Verification items for the finished model (mm, model axes). Round coordinates to 2 decimals unless told otherwise and drop trailing zeros. Write each loop counter-clockwise with the first axis right and the second up, starting at its lowest first coordinate (ties: lowest second). Pieces come first, ordered by that corner, then holes. Notation, with made-up numbers: (12.5, -36.75) -> (42.5, -36.75) arc R14 cw to (42.5, -14.75) -> close; hole circle Ø11 at (-14.5, -2). An arc over 180 degrees is marked (long way). Use CSV: the item, a comma, the result in double quotes.
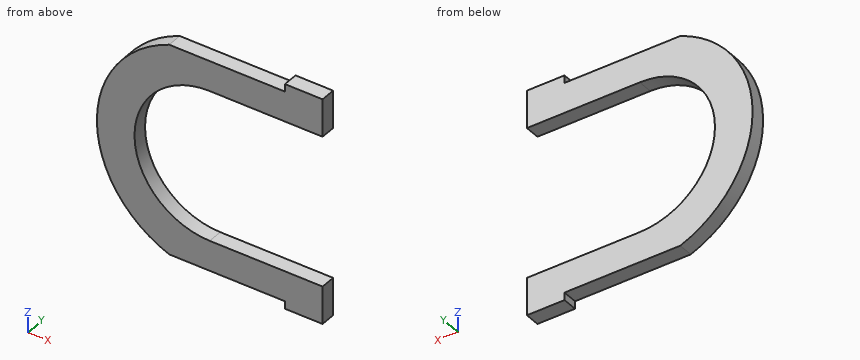
```python
from build123d import *

# Parameters (mm, degrees)
F1_DEPTH = 25.4


with BuildPart() as f1:
    # F0 (on Front) → F1 (new body)
    with BuildSketch(Plane.XZ):
        with BuildLine():
            Line((-68.391593, -177.8), (127, -177.8))
            Line((127, -177.8), (127, -190.5))
            Line((127, -190.5), (190.5, -190.5))
            Line((190.5, -190.5), (190.5, -177.8))
            Line((190.5, -177.8), (190.5, -127))
            Line((190.5, -127), (127, -127))
            Line((127, -127), (0, -127))
            ThreePointArc((0, -127), (-127, 0), (0, 127))
            Line((0, 127), (127, 127))
            Line((127, 127), (190.5, 127))
            Line((190.5, 127), (190.5, 177.8))
            Line((190.5, 177.8), (190.5, 190.5))
            Line((190.5, 190.5), (127, 190.5))
            Line((127, 190.5), (127, 177.8))
            Line((127, 177.8), (-68.391593, 177.8))
            ThreePointArc((-68.391593, 177.8), (-190.5, 0), (-68.391593, -177.8))
        make_face()
    extrude(amount=F1_DEPTH)


solid = f1.part
```
Q1. Section check C-C (z = 0). Record the cut outline in (x, y).
Filled in:
outline,"(-190.5, -25.4) -> (-127, -25.4) -> (-127, 0) -> (-190.5, 0) -> close"
Q2. Section check A-A (x = 122). Record the cut outline in (y, z), plus the area to 3 significant figures.
Filled in:
outline,"(-25.4, -177.8) -> (0, -177.8) -> (0, -127) -> (-25.4, -127) -> close; (-25.4, 127) -> (0, 127) -> (0, 177.8) -> (-25.4, 177.8) -> close"
area,"2,580 mm²"
Q3. Section check D-D (x = -17.5). Record the cut outline in (y, z).
Filled in:
outline,"(-25.4, -177.8) -> (0, -177.8) -> (0, -125.79) -> (-25.4, -125.79) -> close; (-25.4, 125.79) -> (0, 125.79) -> (0, 177.8) -> (-25.4, 177.8) -> close"
Q4. Go/stop test with flat-tipped pins: P1, Ø7.5, axis at x = 60, y = -17.5, coming from the -Z side; P2, Ø6.5, axis at y = -14, z = 186.5, coming from the -X side; P3, Ø3, axis at x = -58.5, y = -13.5, coming from the +Z side. Record where each tip stops, or that it passes through.
Filled in:
P1,"z = -177.8"
P2,"x = 127"
P3,"z = 177.8"
Q5. Material ranges on L1, parallel to Z at x = 157.5, y = -12.25; L2, parallel to Z at x = 0.5, y = -1.25; L3, parallel to X at y = -4, z = -142.5, recorded low to high.
Filled in:
L1,"-190.5 to -127, 127 to 190.5"
L2,"-177.8 to -127, 127 to 177.8"
L3,"-126.43 to 190.5"
Q6. Section check B-B (y = -15.25). Record the cut outline in (x, z).
Filled in:
outline,"(-68.39, -177.8) -> (127, -177.8) -> (127, -190.5) -> (190.5, -190.5) -> (190.5, -127) -> (0, -127) arc R127 cw to (0, 127) -> (190.5, 127) -> (190.5, 190.5) -> (127, 190.5) -> (127, 177.8) -> (-68.39, 177.8) arc R190.5 ccw to start"
